Work out the finished part from the listing and answer in its coordinate system (mm). Face numbers are marked on the shaded views. A direction names the side the tool comes from. Round coordinates to 2 decimals unless told otherwise and drop trailing zeros. Order: outer loops, then holes, each group sorted by start corner. A loop starts at its lowest first (then second) coordinate and runs counter-clockwise, first axis right, second up. Notation, with made-up numbers: (78.5, 59) -> (122.5, 59) arc R19 ccw to (122.5, 95) -> close; hole circle Ø10 at (29, 51.25). An arc over 180 degrees is marked (long way). Use a Markdown table: item, result. Add a question column.
Item 1: Find the intervals of material crossed by L1, parallel to X at y = 0.75, z = 20; L2, parallel to Y at x = 16, z = 19.25; L3, parallel to Y at x = 30, z = 23.5, in increasing order. Write a range as [from, to].
Item 2: A cutting plane is placed at B-B, the plane x = 14. Determine the outline of the cut face in (y, z), plus the area to 3 significant figures.
Item 3: A cutting plane is placed at C-C, the plane y = 6.25. Determine the outline of the cut face in (x, z), plus the area to 3 significant figures.
Item 4: A tool of negligible diameter and unlimited length cuts with its end or side. For the marked faces 4, 5 and 6, from which of +Z, -Z, +X, -X, +Y, -Y can it reach the whole face along a straight path? Write none if from no direction.
Item 5: A cutting plane is placed at A-A, the plane z = 21.25. Determine the outline of the cut face in (x, y), plus the area to 3 significant figures.
Item 6: For a pull along X with two mould halves and no side action, classify the marked faces 1, 2 and 3 as +X half, -X half, draft (parallel to the pull), parting line (faces both ways), or undercut.
Item 7: A cutting plane is placed at D-D, the plane x = 3.5. Determine the outline of the cut face in (y, z).
Item 8: Flat-ended cylindrical pins translate along their axes: P1, Ø6, axis at x = 32, z = 12.5, coming from the +Y side; P2, Ø4, axis at x = 19, z = 10, coming from the +Y side; P3, Ø3, axis at y = 6, z = 13, coming from the -X side. Find the tip coordinate at first contact, or state that the pin passes through.
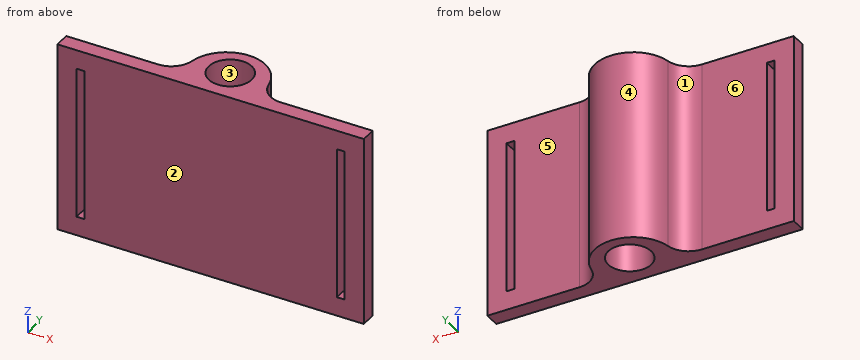
from build123d import *

# Parameters (mm, degrees)
BOSS_EXTRUDE2_DEPTH = 25
SKETCH3_W           = 1
SKETCH3_H           = 20
CUT_EXTRUDE2_DEPTH  = 5
SKETCH4_R           = 2.817174782
CUT_EXTRUDE3_DEPTH  = 36


with BuildPart() as part:
    # Sketch1 → Boss-Extrude2 (new body)
    with BuildSketch(Plane.XY):
        with BuildLine():
            Line((-4.122666018, 0), (-4.122666018, 2))
            Line((-4.122666018, 2), (7.877333982, 2))
            ThreePointArc((7.877333982, 2), (9.83688299, 2.714187595), (10.877333982, 4.521771056))
            ThreePointArc((10.877333982, 4.521771056), (15.877333982, 8.724722816), (20.877333982, 4.521771056))
            ThreePointArc((20.877333982, 4.521771056), (21.917784974, 2.714187595), (23.877333982, 2))
            Line((23.877333982, 2), (35.877333982, 2))
            Line((35.877333982, 2), (35.877333982, 0))
            Line((35.877333982, 0), (-4.122666018, 0))
        make_face()
    extrude(amount=BOSS_EXTRUDE2_DEPTH)

    # Sketch3 → Cut-Extrude2 (cut)
    with BuildSketch(Plane(origin=(0, 0, 0), x_dir=(1, 0, 0), z_dir=(0, 1, 0))):
        with Locations((-1.122666018, -12.5)):
            Rectangle(SKETCH3_W, SKETCH3_H)
        with Locations((32.877333982, -12.5)):
            Rectangle(SKETCH3_W, SKETCH3_H)
    extrude(amount=CUT_EXTRUDE2_DEPTH, mode=Mode.SUBTRACT)

    # Sketch4 → Cut-Extrude3 (cut)
    with BuildSketch(Plane.XY.offset(25)):
        with Locations((15.877333982, 4.5)):
            Circle(SKETCH4_R)
    extrude(amount=-CUT_EXTRUDE3_DEPTH, mode=Mode.SUBTRACT)


solid = part.part
Reported:
| question | item | result |
|---|---|---|
| 1 | L1 | [-4.12, -1.62], [-0.62, 32.38], [33.38, 35.88] |
| 1 | L2 | [0, 1.69], [7.31, 8.72] |
| 1 | L3 | [0, 2] |
| 2 | outline | (0, 0) -> (2.4, 0) -> (2.4, 25) -> (0, 25) -> close; (6.6, 0) -> (8.36, 0) -> (8.36, 25) -> (6.6, 25) -> close |
| 2 | area | 104 mm² |
| 3 | outline | (11.52, 0) -> (13.67, 0) -> (13.67, 25) -> (11.52, 25) -> close; (18.09, 0) -> (20.24, 0) -> (20.24, 25) -> (18.09, 25) -> close |
| 3 | area | 108 mm² |
| 4 | face 4 | +Z, -Z, +Y |
| 4 | face 5 | +Z, -Z, +X, +Y |
| 4 | face 6 | +Z, -Z, -X, +Y |
| 5 | outline | (-4.12, 0) -> (-1.62, 0) -> (-1.62, 2) -> (-4.12, 2) -> close; (-0.62, 0) -> (32.38, 0) -> (32.38, 2) -> (23.88, 2) arc R3.05 cw to (20.88, 4.52) arc R5.08 ccw to (10.88, 4.52) arc R3.05 cw to (7.88, 2) -> (-0.62, 2) -> close; (33.38, 0) -> (35.88, 0) -> (35.88, 2) -> (33.38, 2) -> close; hole circle Ø5.63 at (15.88, 4.5) |
| 5 | area | 112 mm² |
| 6 | face 1 | -X half |
| 6 | face 2 | draft |
| 6 | face 3 | undercut |
| 7 | outline | (0, 0) -> (2, 0) -> (2, 25) -> (0, 25) -> close |
| 8 | P1 | y = 2 |
| 8 | P2 | y = 8.6 |
| 8 | P3 | x = 10.87 |
